Verification items for the finished model (mm, model axes). Face numbers are marked on the shaded views. A direction names the side the tool comes from. Give positions to 0.01 mm unless a question says otherwise; leave off trailing zeros. Loops run counter-clockwise (first coordinate to the right, second up) from the corner with the lowest first, then second, coordinate; pieces in that order, holes last. Notation, with made-up numbers: (65, 25.25) - (82, 25.25) arc R17 cw to (82, 44.25) - close; hole circle Ø9 at (-27, 58). An arc over 180 degrees is marked (long way). One line per item, written item: value. Start each with the question number.
1. Sectioned sample at A-A (x = 0). Record the cut outline in (y, z), plus the area to 3 significant figures.
2. Sectioned sample at C-C (y = 2.75). Record the cut outline in (x, z).
3. Gauge pin test, flat ends, axial feed: pin 1 (5 mm diameter, centred on x = 8, z = -5.5, fed in from +Y); pin 2 (8 mm diameter, centred on y = 7, z = -2.5, fed in from -X); pin 3 (4.5 mm diameter, centred on x = -7.5, z = -7.5, fed in from +Y); pin 4 (2 mm diameter, centred on x = 5, z = 7, fed in from -Y). Record the tip position at first contact, or that the pin passes through.
4. Sectioned sample at D-D (x = -8.25). Record the cut outline in (y, z), plus the area to 3 significant figures.
5. Mould release check, pull along X, two halves, no side actions. Record for the marked faces 4, 5 and 6: pulls with the +X half, pulls with the -X half, needs draft (parallel to the pull), parting line crosses it, or undercut.
6. Scan lines: L1, parallel to X at y = 1.6, z = 7.5; L2, parallel to Y at x = 7, z = -3.5. Record each from-to range of solid material in increasing order. Write a range as [from, to].
7. Access from +Z, -Z, +X, -X, +Y, -Y to the whole of each face (thin tool, end or side, straight path). Record for the marked faces 1, 2 and 3.
8. Sectioned sample at B-B (z = 7.5). Record the cut outline in (x, y), plus the area to 3 significant figures.
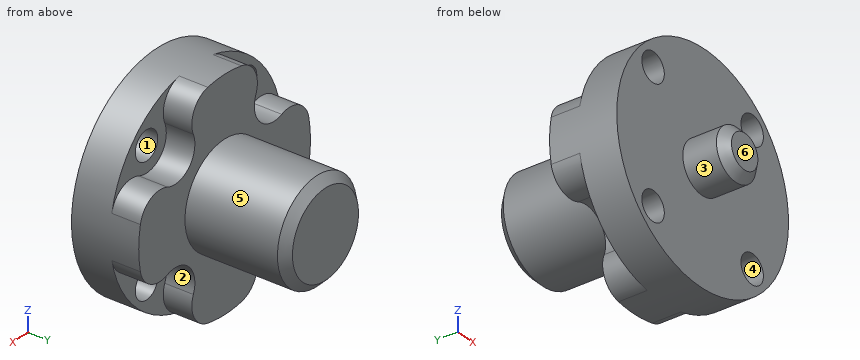
from build123d import *

# Parameters (mm, degrees)
SKETCH1_R                                            = 6
BOSS_EXTRUDE1_DEPTH                                  = 20
SKETCH3_R                                            = 13
BOSS_EXTRUDE2_DEPTH                                  = 8
CBORE_FOR_M3_HEXAGON_SOCKET_HEAD_CAP_SCR_D           = 3.4
CBORE_FOR_M3_HEXAGON_SOCKET_HEAD_CAP_SCR_CBORE_D     = 6
CBORE_FOR_M3_HEXAGON_SOCKET_HEAD_CAP_SCR_CBORE_DEPTH = 3.4
FILLET1_R                                            = 3
CHAMFER1_SIZE                                        = 1
SKETCH7_R                                            = 3
BOSS_EXTRUDE3_DEPTH                                  = 5
CHAMFER2_SIZE                                        = 1


with BuildPart() as part:
    # Sketch1 → Boss-Extrude1 (new body)
    with BuildSketch(Plane(origin=(0, 0, 0), x_dir=(1, 0, 0), z_dir=(0, 1, 0))):
        with Locations(Location((0, 0, 0), (0, 0, 270))):
            Circle(SKETCH1_R)
    extrude(amount=BOSS_EXTRUDE1_DEPTH)

    # Sketch3 → Boss-Extrude2 (add)
    with BuildSketch(Plane.XZ):
        with Locations(Location((0, 0, 0), (0, 0, 270))):
            Circle(SKETCH3_R)
    extrude(amount=-BOSS_EXTRUDE2_DEPTH)

    # CBORE for M3 Hexagon socket head cap screws1 (through all)
    with Locations(Plane(origin=(0, 8, 0), x_dir=(1, 0, 0), z_dir=(0, 1, 0))):
        with Locations((-7.5, 7.5), (-7.5, -7.5), (7.5, -7.5), (7.5, 7.5)):
            CounterBoreHole(CBORE_FOR_M3_HEXAGON_SOCKET_HEAD_CAP_SCR_D / 2, CBORE_FOR_M3_HEXAGON_SOCKET_HEAD_CAP_SCR_CBORE_D / 2, CBORE_FOR_M3_HEXAGON_SOCKET_HEAD_CAP_SCR_CBORE_DEPTH)

    # Fillet1
    fillet1_edges = [part.edges().sort_by_distance(p)[0] for p in [
        (10.495089529, 6.3, -7.671577138),
        (7.671577138, 6.3, -10.495089529),
        (7.671577138, 6.3, 10.495089529),
        (10.495089529, 6.3, 7.671577138),
        (-7.671577138, 6.3, 10.495089529),
        (-10.495089529, 6.3, 7.671577138),
        (-7.671577138, 6.3, -10.495089529),
        (-10.495089529, 6.3, -7.671577138),
    ]]
    fillet(fillet1_edges, radius=FILLET1_R)

    # Chamfer1
    chamfer1_edges = [part.edges().sort_by_distance(p)[0] for p in [
        (0, 20, -6),
    ]]
    chamfer(chamfer1_edges, length=CHAMFER1_SIZE)

    # Sketch7 → Boss-Extrude3 (add)
    with BuildSketch(Plane.XZ):
        with Locations(Location((0, 0, 0), (0, 0, 90))):
            Circle(SKETCH7_R)
    extrude(amount=BOSS_EXTRUDE3_DEPTH)

    # Chamfer2
    chamfer2_edges = [part.edges().sort_by_distance(p)[0] for p in [
        (0, -5, -3),
    ]]
    chamfer(chamfer2_edges, length=CHAMFER2_SIZE)


solid = part.part
Results are:
1. outline: (-5, -2) - (-4, -3) - (0, -3) - (0, -13) - (8, -13) - (8, -6) - (19, -6) - (20, -5) - (20, 5) - (19, 6) - (8, 6) - (8, 13) - (0, 13) - (0, 3) - (-4, 3) - (-5, 2) - close
1. area: 380 mm^2
2. outline: circle Ø26 at (0, 0); hole circle Ø3.4 at (-7.5, -7.5); hole circle Ø3.4 at (-7.5, 7.5); hole circle Ø3.4 at (7.5, -7.5); hole circle Ø3.4 at (7.5, 7.5)
3. pin 1: stops at y = 8
3. pin 2: stops at x = -13
3. pin 3: stops at y = 4.6
3. pin 4: stops at y = 0
4. outline: (0, -10.05) - (4.6, -10.05) - (4.6, -9.03) - (0, -9.03) - close; (0, -5.97) - (4.6, -5.97) - (4.6, -4.6) - (8, -4.6) - (8, 4.6) - (4.6, 4.6) - (4.6, 5.97) - (0, 5.97) - close; (0, 9.03) - (4.6, 9.03) - (4.6, 10.05) - (0, 10.05) - close
4. area: 95.6 mm^2
5. face 4: undercut
5. face 5: parting line crosses it
5. face 6: needs draft
6. L1: x = [-10.62, -9.2], [-5.8, 5.8], [9.2, 10.62]
6. L2: y = [0, 8]
7. face 1: +Y, -Y
7. face 2: +Y
7. face 3: -Y
8. outline: (-10.62, 0) - (-9.2, 0) - (-9.2, 4.6) - (-10.62, 4.6) - close; (-5.8, 0) - (5.8, 0) - (5.8, 4.6) - (4.5, 4.6) - (4.5, 8) - (-4.5, 8) - (-4.5, 4.6) - (-5.8, 4.6) - close; (9.2, 0) - (10.62, 0) - (10.62, 4.6) - (9.2, 4.6) - close
8. area: 97.0 mm^2
